Design review of the part shown in the three views and the two pictorial views. Dimensions are in mm from the part's minimum x, y and z. A direction names the side the tool comes from. Round coordinates to 2 decimals unless told otherwise and drop trailing zeros. Write each loop counter-clockwise with the first axis right and the second up, starting at its lowest first coordinate (ties: lowest second). Pieces come first, ordered by that corner, then holes. Notation, with made-up numbers: (-6.75, 41.5) -> (-1.75, 41.5) arc R16 ccw to (-1.75, 55.5) -> close; hole circle Ø11 at (14, 82). An arc over 180 degrees is marked (long way). One line per question, with ' | ' between items. Start each with the question number.
1) Mouldability with a two-part tool opening along Z and no side actions: class the marked faces 4, 5 and 6 as +Z half, -Z half, draft (parallel to the pull), parting line (faces both ways), or undercut.
2) Consider section A-A (z = 5). Give the boundary of the cut face in (x, y), then the cut area to 3 significant figures.
3) For the marked faces 1, 2 and 3, list the 3-axis set-ups (+Z, -Z, +X, -X, +Y, -Y) from which the entire face can be reached by the end or side of a thin tool; tool diameter is ignored.
4) Consider section C-C (y = 1). Give the boundary of the cut face in (x, z), then the cut area to 3 significant figures.
5) Consider section B-B (x = 5). Give the boundary of the cut face in (y, z).
6) Consider section D-D (y = 4.75). Give the boundary of the cut face in (x, z).
7) Insertion check: pin 1 Ø1.3 at (x, z) = (3.1, 1.71) entering from -Y; pin 2 Ø2 at (x, z) = (3.1, 1.71) entering from -Y; pin 3 Ø0.7 at (x, z) = (3, 2) entering from +Y; pin 4 Ø1 at (y, z) = (4, 6.5) entering from +X. Each pin has a flat end and moves straight along its axis. Give the tip position at first contact, or say it passes through.
8) For probe 1 along X at (y, z) = (1.5, 5); probe 2 along X at (y, z) = (6, 5); probe 3 along Z at (x, y) = (5.25, 6.75), list the stretches that pass through material, from the lowest coordinate up.
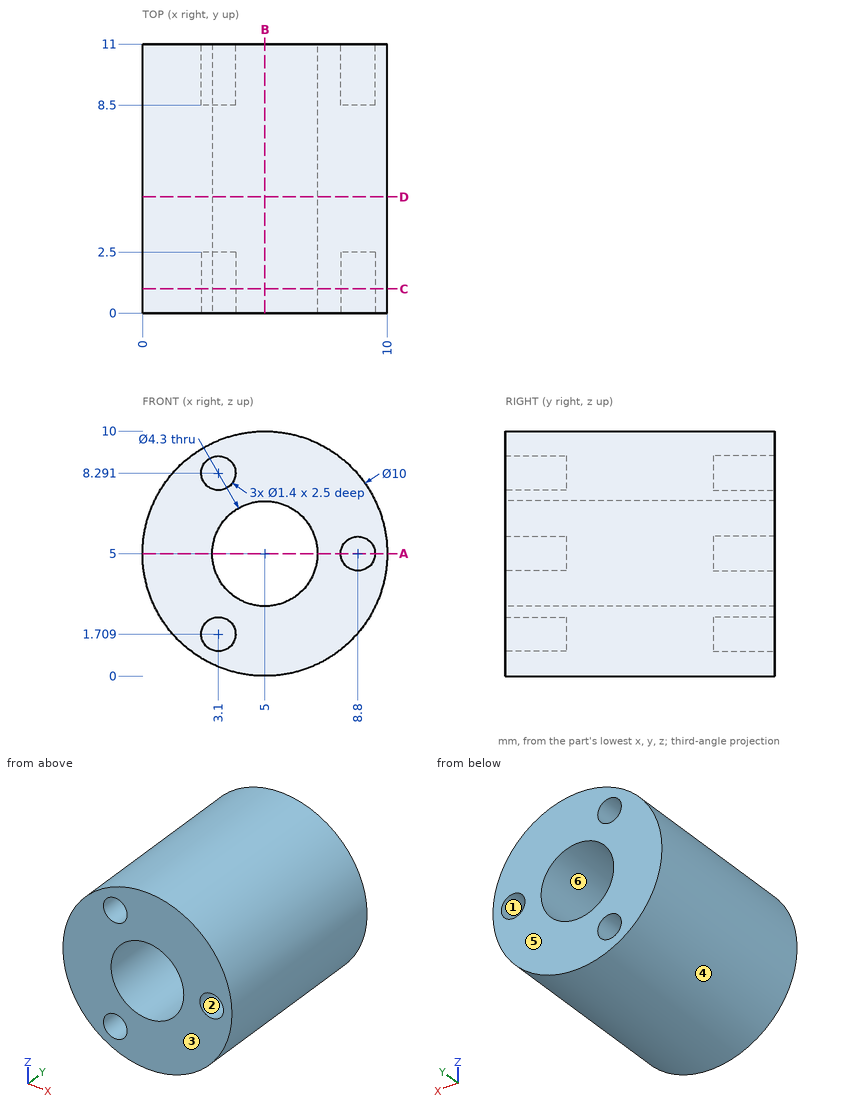
From the geometry:
1) face 4: parting line | face 5: draft | face 6: undercut
2) outline: (0, 0) -> (2.85, 0) -> (2.85, 11) -> (0, 11) -> close; (7.15, 0) -> (8.1, 0) -> (8.1, 2.5) -> (9.5, 2.5) -> (9.5, 0) -> (10, 0) -> (10, 11) -> (9.5, 11) -> (9.5, 8.5) -> (8.1, 8.5) -> (8.1, 11) -> (7.15, 11) -> close | area: 55.7 mm2
3) face 1: +Y | face 2: -Y | face 3: +Z, -Z, +X, -X, -Y
4) outline: circle Ø10 at (5, 5); hole circle Ø1.4 at (3.1, 1.71); hole circle Ø1.4 at (3.1, 8.29); hole circle Ø4.3 at (5, 5); hole circle Ø1.4 at (8.8, 5) | area: 59.4 mm2
5) outline: (0, 0) -> (11, 0) -> (11, 2.85) -> (0, 2.85) -> close; (0, 7.15) -> (11, 7.15) -> (11, 10) -> (0, 10) -> close
6) outline: circle Ø10 at (5, 5); hole circle Ø4.3 at (5, 5)
7) pin 1: stops at y = 2.5 | pin 2: stops at y = 0 | pin 3: stops at y = 8.5 | pin 4: stops at x = 9.9
8) probe 1: x = 0 to 2.85, 7.15 to 8.1, 9.5 to 10 | probe 2: x = 0 to 2.85, 7.15 to 10 | probe 3: z = 0.01 to 2.86, 7.14 to 9.99
